Geometry: see drawing. Coordinates: mm, zero at the bounding-box minimum. A direction names the side the tool comes from. Give positions to 0.01 mm unless a question says otherwise; leave off trailing zeros. Write each loop counter-clockwise with the first axis right and the second up, starting at its lowest first coordinate (ties: lowest second). Pieces come first, ordered by that corner, then holes.
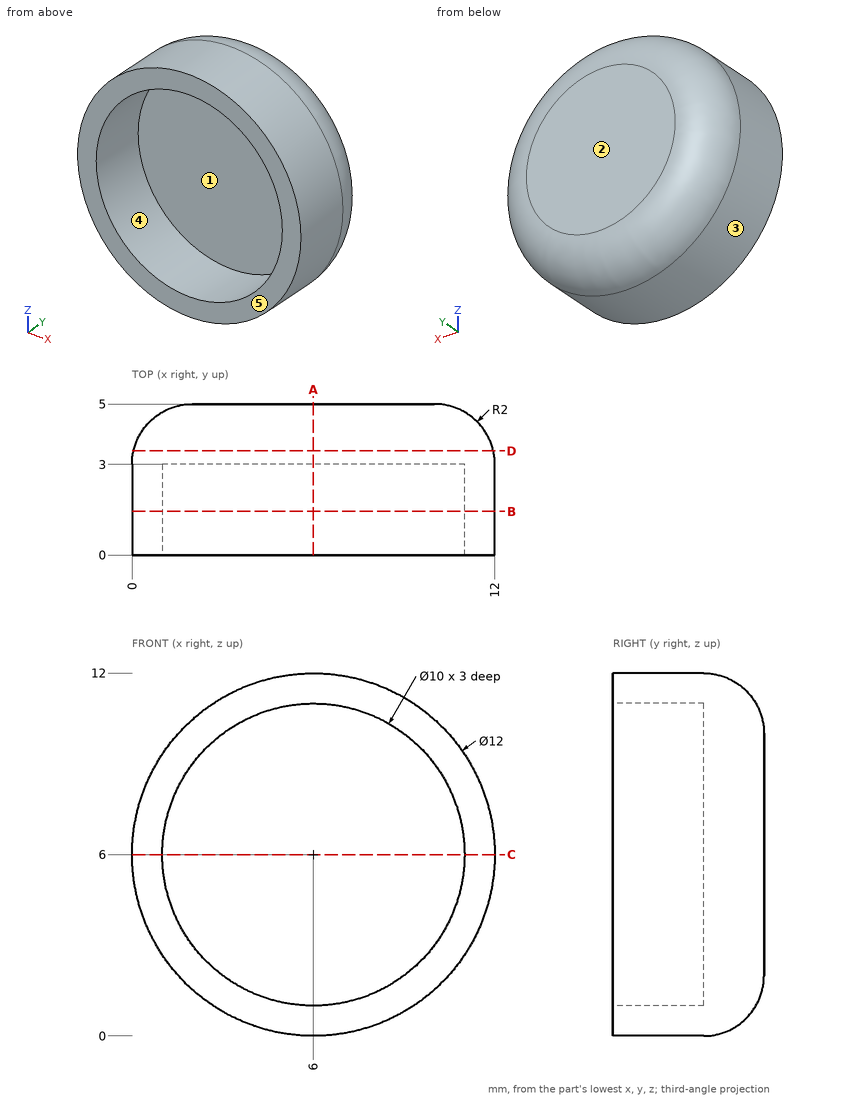
Q1. Section B-B, the plane y = 1.45. Return the cut outline in (x, z), then the cut area to 3 significant figures.
Q2. Section C-C, the plane z = 6. Return the cut outline in (x, y).
Q3. Section A-A, the plane x = 6. Return the cut outline in (y, z).
Q4. Section D-D, the plane y = 3.45. Return the cut outline in (x, z).
Q5. Mould query, pull axis Z, two halves, no side actions, for the marked faces 3, 4 and 5. Classes: +Z half, -Z half, draft (parallel to the pull), parting line (faces both ways), or undercut.
Q6. Material intervals for line 1 along Z through (x, y) = (6, 0.8); line 2 along Z through (x, y) = (2.5, 2.1), sorted ascending.
Q7. Access query for the marked faces 1 and 2. Directions: +Z, -Z, +X, -X, +Y, -Y. A direction counts if a zero-diameter tool reaches every point of the face in a straight line with its end or side. Return the directions, or none.
Q8. Pin query (flat end, axial travel): pin 1 (3 mm diameter, centred on x = 5.5, z = 4.5, fed in from -Y); pin 2 (1.5 mm diameter, centred on y = 4, z = 4, fed in from +X); pin 3 (1.5 mm diameter, centred on x = 6, y = 4.5, fed in from -Z); pin 4 (3 mm diameter, centred on y = 2, z = 6.5, fed in from +X). Return the tip coordinate at first contact, or that it passes through.
Solutions:
1. outline: circle Ø12 at (6, 6); hole circle Ø10 at (6, 6)
1. area: 34.6 mm2
2. outline: (0, 0) - (1, 0) - (1, 3) - (11, 3) - (11, 0) - (12, 0) - (12, 3) arc R2 ccw to (10, 5) - (2, 5) arc R2 ccw to (0, 3) - close
3. outline: (0, 0) - (3, 0) arc R2 ccw to (5, 2) - (5, 10) arc R2 ccw to (3, 12) - (0, 12) - (0, 11) - (3, 11) - (3, 1) - (0, 1) - close
4. outline: circle Ø11.9 at (6, 6)
5. face 3: parting line
5. face 4: undercut
5. face 5: draft
6. line 1: z = 0 to 1, 11 to 12
6. line 2: z = 1.13 to 2.43, 9.57 to 10.87
7. face 1: -Y
7. face 2: +Z, -Z, +X, -X, +Y
8. pin 1: stops at y = 3
8. pin 2: stops at x = 11.76
8. pin 3: stops at z = 0.15
8. pin 4: stops at x = 12
